Read the model definition and answer for the solid it produces. Units are mm, in the model's axes. A direction names the side the tool comes from. Give positions to 0.01 mm unless a question says otherwise; leave off trailing zeros. Order: outer loops, then holes, each group sorted by start corner. A loop starts at its lowest first (then second) coordinate and runs counter-clockwise, first axis right, second up. Notation, with made-up numbers: (4.5, 52) -> (39.5, 52) arc R10 cw to (39.5, 56) -> close; hole circle Ø11 at (-21.5, -9). An arc over 180 degrees is marked (long way). Use one line per item in the form item = value.
```python
from build123d import *

# Parameters (mm, degrees)
BOSS_EXTRUDE2_DEPTH = 50.8
SKETCH4_R           = 3.175
CUT_EXTRUDE1_DEPTH  = 45.45
SKETCH5_R           = 3.175
CUT_EXTRUDE2_DEPTH  = 4.175


with BuildPart() as part:
    # Sketch3 → Boss-Extrude2 (new body)
    with BuildSketch(Plane.XY):
        Polygon((0, 0), (63.5, 0), (63.5, 3.175), (44.45, 3.175), (44.45, 28.575), (41.275, 28.575), (41.275, 3.175), (22.225, 3.175), (22.225, 28.575), (19.05, 28.575), (19.05, 3.175), (0, 3.175), align=None)
    extrude(amount=BOSS_EXTRUDE2_DEPTH)

    # Sketch4 → Cut-Extrude1 (cut, through all)
    with BuildSketch(Plane.ZY.offset(-19.05)):
        with Locations((12.7, 15.875)):
            Circle(SKETCH4_R)
        with Locations((38.1, 15.875)):
            Circle(SKETCH4_R)
    extrude(amount=-CUT_EXTRUDE1_DEPTH, mode=Mode.SUBTRACT)

    # Sketch5 → Cut-Extrude2 (cut, through all)
    with BuildSketch(Plane(origin=(0, 3.175, 0), x_dir=(1, 0, 0), z_dir=(0, 1, 0))):
        with Locations((9.525, -38.1)):
            Circle(SKETCH5_R)
        with Locations((9.525, -12.7)):
            Circle(SKETCH5_R)
        with Locations((53.975, -12.7)):
            Circle(SKETCH5_R)
        with Locations((53.975, -38.1)):
            Circle(SKETCH5_R)
    extrude(amount=-CUT_EXTRUDE2_DEPTH, mode=Mode.SUBTRACT)


solid = part.part
```
Item 1: The part is cut by section D-D on x = 55.5. Give the vertices of the cut face in (y, z) (3 decimals).
Checks:
outline = (0, 0) -> (3.175, 0) -> (3.175, 9.915) -> (0, 9.915) -> close; (0, 15.485) -> (3.175, 15.485) -> (3.175, 35.315) -> (0, 35.315) -> close; (0, 40.885) -> (3.175, 40.885) -> (3.175, 50.8) -> (0, 50.8) -> close
Item 2: Given pin 1 Ø4 at (x, z) = (53.975, 38.1) entering from -Y; pin 2 Ø9.5 at (x, z) = (13.5, 32.5) entering from +Y (3 decimals); pin 3 Ø7.5 at (y, z) = (15.875, 38.1) entering from -X; pin 4 Ø7.5 at (y, z) = (15.875, 38.1) entering from +X, each flat-ended and moving along its own axis, determine where each tip first touches the part or whether it passes through.
Checks:
pin_1 = through
pin_2 = 3.175
pin_3 = 19.05
pin_4 = 44.45
Item 3: The part is cut by section A-A on y = 2. Give the vertices of the cut face in (x, z) (3 decimals).
Checks:
outline = (0, 0) -> (63.5, 0) -> (63.5, 50.8) -> (0, 50.8) -> close; hole circle Ø6.35 at (9.525, 12.7); hole circle Ø6.35 at (9.525, 38.1); hole circle Ø6.35 at (53.975, 12.7); hole circle Ø6.35 at (53.975, 38.1)
Item 4: Straight lines are drawn through the part: L1, parallel to X at y = 0.8, z = 38.1; L2, parallel to X at y = 14.5, z = 33 (3 decimals); L3, parallel to Y at x = 32, z = 40 (3 decimals). For each, find the intervals that lie inside material, in ascending order. Write a range as from..to.
Checks:
L1 = 0..6.35, 12.7..50.8, 57.15..63.5
L2 = 19.05..22.225, 41.275..44.45
L3 = 0..3.175
Item 5: Which of the six approach directions +Z, -Z, +X, -X, +Y, -Y give full straight-line access (tool end or side, diameter ignored) to faces 1 (the flat face through (44.45, 16, 25)), 2 (the flat face through (41.275, 16, 25)), 3 (the flat face through (10, 3.175, 25))?
Checks:
face_1 = +Z, -Z, +X, +Y
face_2 = +Z, -Z, +Y
face_3 = +Z, -Z, -X, +Y
Item 6: The part is cut by section C-C on y = 22.25. Give the vertices of the cut face in (x, z) (3 decimals).
Checks:
outline = (19.05, 0) -> (22.225, 0) -> (22.225, 50.8) -> (19.05, 50.8) -> close; (41.275, 0) -> (44.45, 0) -> (44.45, 50.8) -> (41.275, 50.8) -> close
Item 7: The part is cut by section B-B on z = 38.1. Give the vertices of the cut face in (x, y) (3 decimals).
Checks:
outline = (0, 0) -> (6.35, 0) -> (6.35, 3.175) -> (0, 3.175) -> close; (12.7, 0) -> (50.8, 0) -> (50.8, 3.175) -> (44.45, 3.175) -> (44.45, 12.7) -> (41.275, 12.7) -> (41.275, 3.175) -> (22.225, 3.175) -> (22.225, 12.7) -> (19.05, 12.7) -> (19.05, 3.175) -> (12.7, 3.175) -> close; (19.05, 19.05) -> (22.225, 19.05) -> (22.225, 28.575) -> (19.05, 28.575) -> close; (41.275, 19.05) -> (44.45, 19.05) -> (44.45, 28.575) -> (41.275, 28.575) -> close; (57.15, 0) -> (63.5, 0) -> (63.5, 3.175) -> (57.15, 3.175) -> close
Item 8: Determine the mould class of faces 4 (the flat face through (27, 3, 0)), 5 (the cylindrical face through (20.615, 16.015, 34.928)), 6 (the flat face through (0, 2, 25)) for opening direction Z: +Z half, -Z half, draft (parallel to the pull), parting line (faces both ways), or undercut.
Checks:
face_4 = -Z half
face_5 = undercut
face_6 = draft
